Read the model definition and answer for the solid it produces. Units are mm, in the model's axes. Face numbers are marked on the shaded views. A direction names the side the tool comes from. Round coordinates to 2 decimals unless told otherwise and drop trailing zeros. Order: outer loops, then holes, each group sorted by start corner. A loop starts at its lowest first (then second) coordinate and runs counter-clockwise, first axis right, second up. Notation, with made-up numbers: (-35.5, 42) - (-30.5, 42) arc R14 ccw to (-30.5, 60) - close; hole circle Ø3 at (-28.5, 13). An arc over 180 degrees is marked (long way). Answer as a JSON object with one key per item and string values. Group by question number.
Q1. Consider line 1 (Z direction, x = 6, y = -30); line 2 (Y direction, x = 8.25, z = 16); line 3 (X direction, y = -13, z = 26.75). Determine where each line is inside the solid, lowest interval first.
Q2. A cutting plane is placed at A-A on y = -65. Determine the outline of the cut face in (x, z).
Q3. A cutting plane is placed at B-B on z = 15. Determine the outline of the cut face in (x, y).
Q4. The mould has two halves that part along X. Classify the marked faces 1, 2 and 3: pulls with the +X half, pulls with the -X half, needs draft (parallel to the pull), parting line crosses it, or undercut.
Q5. A tool of negligible diameter and unlimited length cuts with its end or side. For the marked faces 4 and 5, from which of +Z, -Z, +X, -X, +Y, -Y can it reach the whole face along a straight path? Write none if from no direction.
Q6. Given pin 1 Ø6 at (x, y) = (10, -65) entering from +Z; pin 2 Ø6.5 at (y, z) = (-10, 15) entering from +X; pin 3 Ø5 at (x, z) = (14.5, 19.5) entering from +Y; pin 4 Ø4 at (y, z) = (-36.5, 21.5) entering from -X, each flat-ended and moving along its own axis, determine where each tip first touches the part or whether it passes through.
Q7. A cutting plane is placed at C-C on z = 4.5. Determine the outline of the cut face in (x, y), and give its area (3 significant figures).
Q8. A cutting plane is placed at D-D on x = 16.25. Determine the outline of the cut face in (y, z).
```python
from build123d import *

# Parameters (mm, degrees)
F1_DEPTH = 30
F3_D     = 10
F5_D     = 5
F7_D     = 5
F8_R     = 2
F9_R     = 1


with BuildPart() as f1:
    # F0 (on Top) → F1 (new body)
    with BuildSketch(Plane.XY):
        Polygon((10, 0), (0, 0), (0, -75), (20, -75), (20, -55), (10, -55), align=None)
    extrude(amount=F1_DEPTH)

    # F3 (through all)
    with Locations(Plane.XY.offset(30)):
        with Locations((10, -65)):
            Hole(F3_D / 2)

    # F5 (through all)
    with Locations(Plane.YZ.offset(10)):
        with Locations((-10, 15)):
            Hole(F5_D / 2)

    # F7 (through all)
    with Locations(Plane.YZ.offset(10)):
        with Locations((-30, 15)):
            Hole(F7_D / 2)

    # F8
    f8_edges = [f1.edges().sort_by_distance(p)[0] for p in [
        (10, 0, 15),
        (20, -55, 15),
        (10, -55, 15),
        (20, -75, 15),
    ]]
    fillet(f8_edges, radius=F8_R)

    # F9
    f9_edges = [f1.edges().sort_by_distance(p)[0] for p in [
        (4, 0, 30),
        (10, -27.5, 0),
    ]]
    fillet(f9_edges, radius=F9_R)


solid = f1.part
```
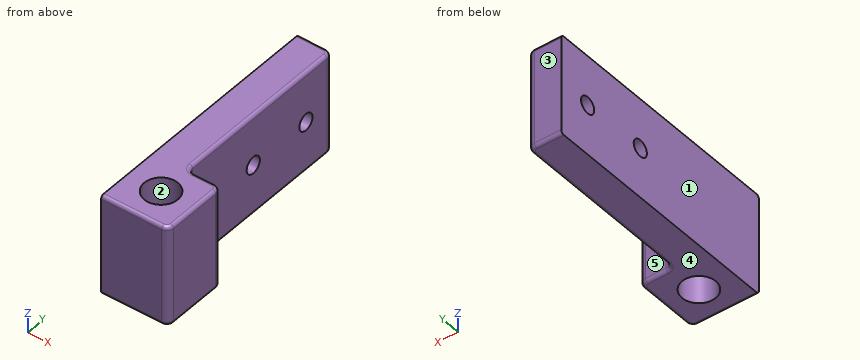
Result set:
{
 "1": {"line 1": "z = 0 to 12.5, 17.5 to 30", "line 2": "y = -75 to -69.68, -60.32 to -32.29, -27.71 to -12.29, -7.71 to -0.02", "line 3": "x = 0 to 10"},
 "2": {"outline": "(0, 0) - (5, 0) - (5, 30) - (0, 30) - close; (15, 0) - (19, 0) arc R1 ccw to (20, 1) - (20, 29) arc R1 ccw to (19, 30) - (15, 30) - close"},
 "3": {"outline": "(0, -75) - (18, -75) arc R2 ccw to (20, -73) - (20, -57) arc R2 ccw to (18, -55) - (12, -55) arc R2 cw to (10, -53) - (10, -32.5) - (0, -32.5) - close; (0, -27.5) - (10, -27.5) - (10, -12.5) - (0, -12.5) - close; (0, -7.5) - (10, -7.5) - (10, -2) arc R2 ccw to (8, 0) - (0, 0) - close; hole circle Ø10 at (10, -65)"},
 "4": {"face 1": "pulls with the -X half", "face 2": "undercut", "face 3": "needs draft"},
 "5": {"face 4": "-Z, +X, -X, +Y, -Y", "face 5": "+Z, -Z, +X, +Y"},
 "6": {"pin 1": "passes through", "pin 2": "stops at x = 10", "pin 3": "stops at y = -55", "pin 4": "stops at x = 0"},
 "7": {"outline": "(0, -75) - (18, -75) arc R2 ccw to (20, -73) - (20, -57) arc R2 ccw to (18, -55) - (12, -55) arc R2 cw to (10, -53) - (10, -2) arc R2 ccw to (8, 0) - (0, 0) - close; hole circle Ø10 at (10, -65)", "area": "870 mm²"},
 "8": {"outline": "(-75, 1) arc R1 ccw to (-74, 0) - (-56, 0) arc R1 ccw to (-55, 1) - (-55, 29) arc R1 ccw to (-56, 30) - (-74, 30) arc R1 ccw to (-75, 29) - close"}
}
